Can you work these out from the drawing? Everything is in mm from the part's minimum corner. A direction names the side the tool comes from. Coordinates: 2 decimals unless noted, no trailing zeros. Order: outer loops, then holes, each group sorted by start corner. A loop starts at its lowest first (then second) coordinate and runs counter-clockwise, first axis right, second up. Notation, with made-up numbers: (-15.75, -1) - (-5.75, -1) arc R16 cw to (-5.75, 7) - close; hole circle Ø7 at (16.5, 45). An arc over 180 degrees is marked (long way). Answer as CSV lines item,"result". Start each with the question number.
Q1. For the marked faces 1 and 2, which set-ups out of +Z, -Z, +X, -X, +Y, -Y let a thin tool reach every point of the face, with its end or its side?
Q2. Suppose I cut it at C-C (y = 0.4). Please give me the cut outline in (x, z).
Q3. For pin 1 Ø1.5 at (x, y) = (3, 2.5) entering from +Z; pin 2 Ø3 at (x, z) = (7.5, 4.5) entering from -Y, each with a flat end and sliding along its axis, tell me the tip position at first contact or that it passes through.
Q4. Suppose I cut it at B-B (x = 7.5). Please give me the cut outline in (y, z).
Q5. I need wall thicknesses on line 1 (Z direction, x = 1.75, y = 2.1); line 2 (X direction, y = 1.9, z = 3.55); line 3 (Y direction, x = 6.75, z = 4.25). Which ranges of each line are inside material? Lowest first, please.
Q6. Suppose I cut it at A-A (z = 1.2). Please give me the cut outline in (x, y), then the cut area to 3 significant figures.
Q7. Suppose I cut it at D-D (z = 3.7). Please give me the cut outline in (x, y), then the cut area to 3 significant figures.
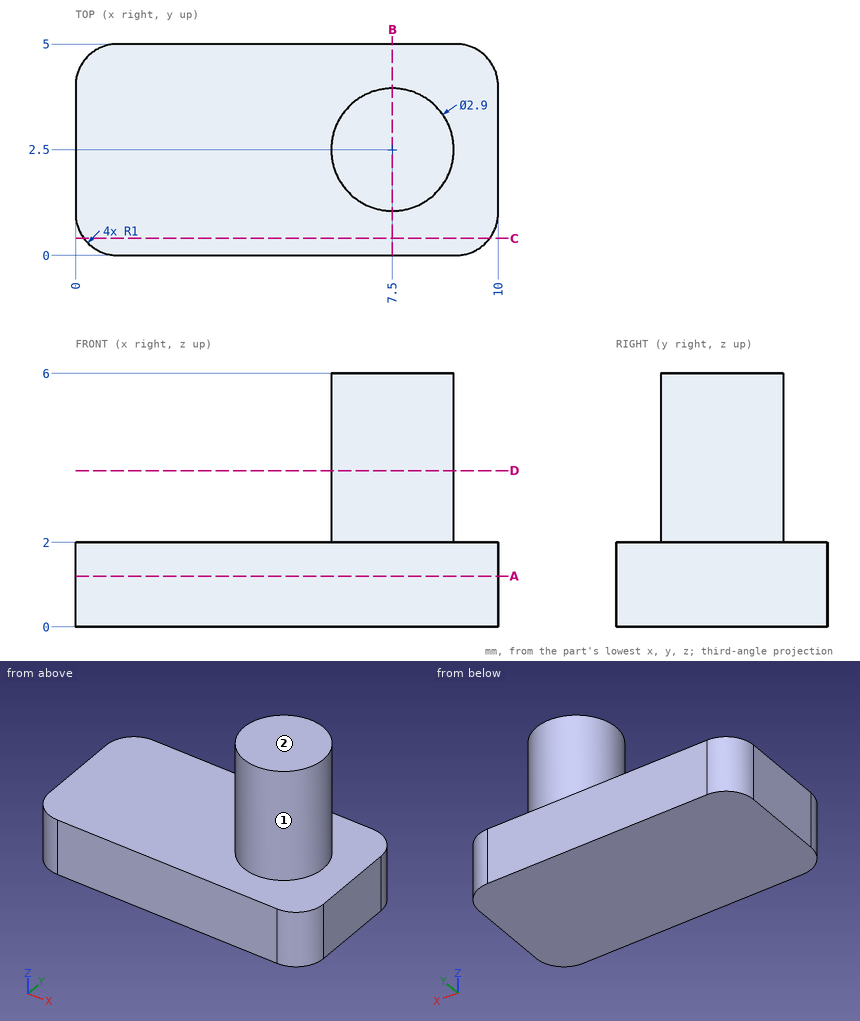
Here are the results:
1,face 1,"+Z"
1,face 2,"+Z, +X, -X, +Y, -Y"
2,outline,"(0.2, 0) - (9.8, 0) - (9.8, 2) - (0.2, 2) - close"
3,pin 1,"stops at z = 2"
3,pin 2,"stops at y = 1.05"
4,outline,"(0, 0) - (5, 0) - (5, 2) - (3.95, 2) - (3.95, 6) - (1.05, 6) - (1.05, 2) - (0, 2) - close"
5,line 1,"z = 0 to 2"
5,line 2,"x = 6.18 to 8.82"
5,line 3,"y = 1.26 to 3.74"
6,outline,"(0, 1) arc R1 ccw to (1, 0) - (9, 0) arc R1 ccw to (10, 1) - (10, 4) arc R1 ccw to (9, 5) - (1, 5) arc R1 ccw to (0, 4) - close"
6,area,"49.1 mm²"
7,outline,"circle Ø2.9 at (7.5, 2.5)"
7,area,"6.61 mm²"
